Job drawing, mm, ordinate dimensions from the low corner. One solid piece. A direction names the side the tool comes from. Give positions to 0.01 mm unless a question says otherwise; leave off trailing zeros. Order: outer loops, then holes, each group sorted by start corner. A loop starts at its lowest first (then second) coordinate and runs counter-clockwise, first axis right, second up.
Item 1: Band-saw the part on A-A on z = 10.5. Give the cut face in (x, y).
Item 2: Band-saw the part on C-C on x = 8. Give the cut face in (y, z), plus the area to 3 significant figures.
Item 3: Flat gauge pins, fed straight in: P1, Ø4, axis at x = 10, z = 7, coming from the +Y side; P2, Ø3.5, axis at x = 7.5, z = 4.5, coming from the +Y side; P3, Ø2.5, axis at x = 7.5, z = 10.5, coming from the -Y side; P4, Ø2, axis at y = 7, z = 10.5, coming from the +X side. Where does each tip first touch, or does it go through?
Item 4: Which spindle directions (+Z, -Z, +X, -X, +Y, -Y) get a long thin tool onto all of the face, cutting with end or side? Do the marked faces 1 and 2. Say none if no direction does.
Item 5: Band-saw the part on D-D on x = 11.5. Give the cut face in (y, z).
Item 6: Wall check: L1, parallel to Y at x = 1.55, z = 7.5; L2, parallel to Z at x = 7.5, y = 0.4; L3, parallel to Z at x = 7.5, y = 1.4. Give the ranges that are in metal, low to high.
Item 7: Band-saw the part on B-B on y = 22.5. Give the cut face in (x, z).
Item 8: Two-plate mould, pull along Z, no slides. Class the marked faces 3 and 4: released by +Z, released by -Z, zero draft, split by the parting line, or undercut.
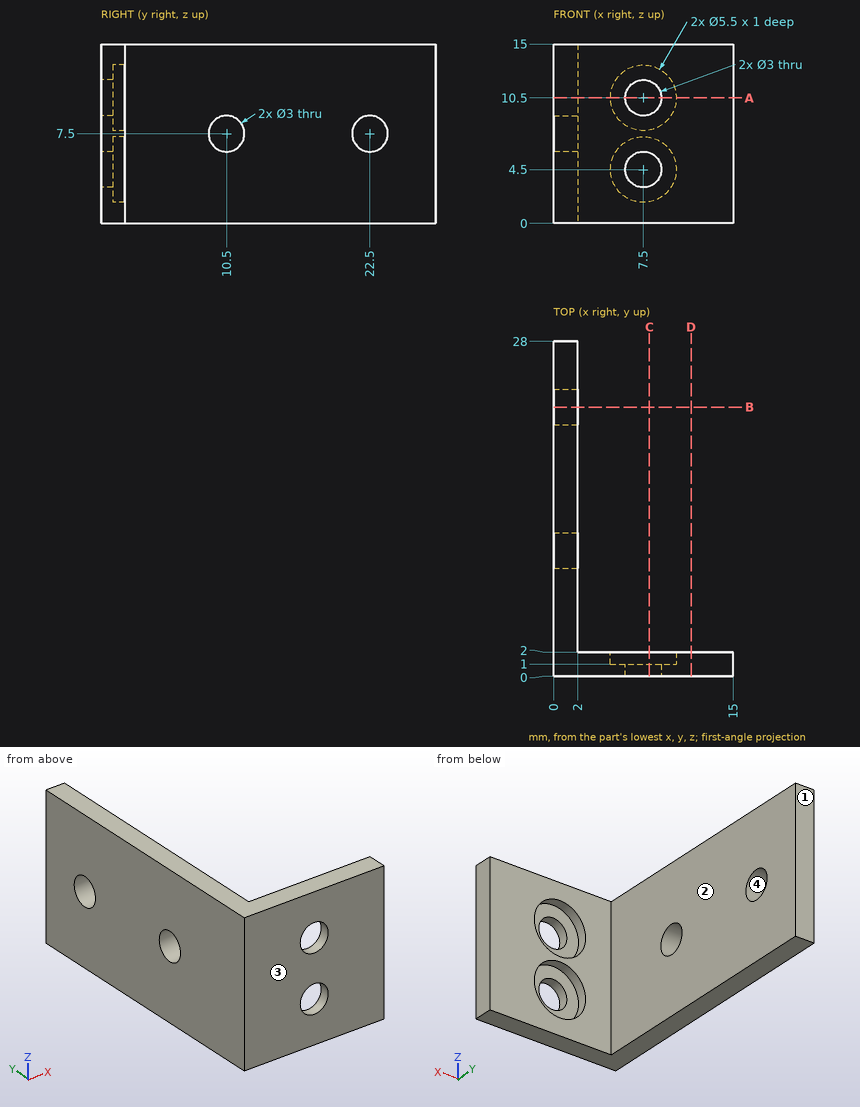
The answers:
1. outline: (0, 0) - (6, 0) - (6, 1) - (4.75, 1) - (4.75, 2) - (2, 2) - (2, 28) - (0, 28) - close; (9, 0) - (15, 0) - (15, 2) - (10.25, 2) - (10.25, 1) - (9, 1) - close
2. outline: (0, 0) - (2, 0) - (2, 1.8) - (1, 1.8) - (1, 3.09) - (0, 3.09) - close; (0, 5.91) - (1, 5.91) - (1, 7.2) - (2, 7.2) - (2, 7.8) - (1, 7.8) - (1, 9.09) - (0, 9.09) - close; (0, 11.91) - (1, 11.91) - (1, 13.2) - (2, 13.2) - (2, 15) - (0, 15) - close
2. area: 13.5 mm2
3. P1: stops at y = 2
3. P2: stops at y = 1
3. P3: passes through
3. P4: stops at x = 2
4. face 1: +Z, -Z, +X, -X, +Y
4. face 2: +Z, -Z, +X, +Y
5. outline: (0, 0) - (2, 0) - (2, 15) - (0, 15) - close
6. L1: y = 0 to 9, 12 to 21, 24 to 28
6. L2: z = 0 to 3, 6 to 9, 12 to 15
6. L3: z = 0 to 1.75, 7.25 to 7.75, 13.25 to 15
7. outline: (0, 0) - (2, 0) - (2, 6) - (0, 6) - close; (0, 9) - (2, 9) - (2, 15) - (0, 15) - close
8. face 3: zero draft
8. face 4: undercut
